The model under review builds one solid part; all positions refer to its coordinate system, in mm. A direction names the side the tool comes from. Give positions to 0.01 mm unless a question says otherwise; leave off trailing zeros. Order: outer loops, then holes, each group sorted by start corner. A loop starts at its lowest first (then second) coordinate and runs counter-clockwise, first axis right, second up. Notation, with made-up numbers: (12, -36.5) -> (20, -36.5) arc R21 cw to (20, -1.5) -> close; hole circle Ø6 at (72, 1). An arc over 180 degrees is marked (long way). Use one line per item in the form item = value.
```python
from build123d import *

# Parameters (mm, degrees)
SKETCH1_W           = 80
SKETCH1_H           = 50
SKETCH1_R           = 2.5
BOSS_EXTRUDE1_DEPTH = 5


with BuildPart() as part:
    # Sketch1 → Boss-Extrude1 (new body)
    with BuildSketch(Plane(origin=(0, 0, 0), x_dir=(1, 0, 0), z_dir=(0, 1, 0))):
        with Locations((40, 25)):
            Rectangle(SKETCH1_W, SKETCH1_H)
        with Locations(Location((55, 25, 0), (0, 0, 270))):
            Circle(SKETCH1_R, mode=Mode.SUBTRACT)
        with BuildLine():
            Line((10, 43), (20, 43))
            ThreePointArc((20, 43), (23, 40), (20, 37))
            Line((20, 37), (10, 37))
            ThreePointArc((10, 37), (7, 40), (10, 43))
        make_face(mode=Mode.SUBTRACT)
        with BuildLine():
            Line((10, 13), (20, 13))
            ThreePointArc((20, 13), (23, 10), (20, 7))
            Line((20, 7), (10, 7))
            ThreePointArc((10, 7), (7, 10), (10, 13))
        make_face(mode=Mode.SUBTRACT)
    extrude(amount=BOSS_EXTRUDE1_DEPTH)


solid = part.part
```
1. The part is to be moulded in two halves that separate along X. For faces 1 (the face through (80, 2, -25)), 2 (the face through (39, 2, -50)), 3 (the face through (23, 2, -10)), say which applies: +X half, -X half, draft (parallel to the pull), parting line (faces both ways), or undercut.
Values:
face_1 = +X half
face_2 = draft
face_3 = undercut
2. Add section B-B on z = -10. Give the boundary of the cut face in (x, y).
Values:
outline = (0, 0) -> (7, 0) -> (7, 5) -> (0, 5) -> close; (23, 0) -> (80, 0) -> (80, 5) -> (23, 5) -> close
3. Tool access review of faces 4 (the face through (39, 5, -25)), 5 (the face through (15, 2, -13)): name each direction out of +Z, -Z, +X, -X, +Y, -Y from which nothing blocks a thin tool from reaching the whole face with its end or side.
Values:
face_4 = +Z, -Z, +X, -X, +Y
face_5 = +Y, -Y
4. Add section A-A on x = 55. Give the boundary of the cut face in (y, z), then the cut area to 3 significant figures.
Values:
outline = (0, -50) -> (5, -50) -> (5, -27.5) -> (0, -27.5) -> close; (0, -22.5) -> (5, -22.5) -> (5, 0) -> (0, 0) -> close
area = 225 mm^2
5. Add section C-C on y = 1.15. Give the boundary of the cut face in (x, z), then the cut area to 3 significant figures.
Values:
outline = (0, -50) -> (80, -50) -> (80, 0) -> (0, 0) -> close; hole (10, -43) -> (20, -43) arc R3 ccw to (20, -37) -> (10, -37) arc R3 ccw to start; hole (10, -13) -> (20, -13) arc R3 ccw to (20, -7) -> (10, -7) arc R3 ccw to start; hole circle Ø5 at (55, -25)
area = 3,800 mm^2
6. Add section D-D on x = 14. Give the boundary of the cut face in (y, z).
Values:
outline = (0, -50) -> (5, -50) -> (5, -43) -> (0, -43) -> close; (0, -37) -> (5, -37) -> (5, -13) -> (0, -13) -> close; (0, -7) -> (5, -7) -> (5, 0) -> (0, 0) -> close
7. For L1, parallel to Z at x = 11, y = 2.7; L2, parallel to X at y = 2, z = -10; L3, parallel to X at y = 3.55, z = -25, list the stretches that pass through material, from the lowest coordinate up.
Values:
L1 = -50 to -43, -37 to -13, -7 to 0
L2 = 0 to 7, 23 to 80
L3 = 0 to 52.5, 57.5 to 80
